```python
from build123d import *

# Parameters (mm, degrees)
BOSS_EXTRU_1_OUTLINE_R = 5
BOSS_EXTRU_1_DEPTH     = 5
CONG_2_R               = 10
CONG_3_R               = 5


# Read off the part's stored shape, not the designer's step: Boss.-Extru.1
with BuildPart() as part:
    # Boss.-Extru.1 outline → Boss.-Extru.1 (new body)
    with BuildSketch(Plane.XY):
        with BuildLine():
            Line((111.825417275, 56.670302216), (105.808192277, 57.923261539))
            ThreePointArc((105.808192277, 57.923261539), (103.288971945, 61.767546768), (107.133257174, 64.2867671))
            Line((107.133257174, 64.2867671), (113.037155155, 63.057405721))
            Line((113.037155155, 63.057405721), (115.346853986, 64.014114302))
            Line((115.346853986, 64.014114302), (111.520019662, 73.252909628))
            Line((111.520019662, 73.252909628), (91.607534943, 56.252195883))
            Line((91.607534943, 56.252195883), (84.536467131, 63.323263695))
            Line((84.536467131, 63.323263695), (82.768700178, 61.555496742))
            Line((82.768700178, 61.555496742), (81.64515805, 55.630550004))
            ThreePointArc((81.64515805, 55.630550004), (77.846557681, 53.042957448), (75.258965125, 56.841557817))
            Line((75.258965125, 56.841557817), (76.404073966, 62.880235609))
            Line((76.404073966, 62.880235609), (59.03555307, 80.248756505))
            Line((59.03555307, 80.248756505), (63.323263695, 84.536467131))
            Line((63.323263695, 84.536467131), (56.252195883, 91.607534943))
            ThreePointArc((56.252195883, 91.607534943), (41.138468979, 99.317049745), (25, 104.552618332))
            Line((25, 104.552618332), (15, 104.552618332))
            Line((15, 104.552618332), (15, 102.052618332))
            Line((15, 102.052618332), (18.395105759, 97.068584057))
            ThreePointArc((18.395105759, 97.068584057), (17.538793922, 92.552863734), (13.023073599, 93.40917557))
            Line((13.023073599, 93.40917557), (9.56279781, 98.488879813))
            Line((9.56279781, 98.488879813), (-15, 98.488879813))
            Line((-15, 98.488879813), (-15, 104.552618332))
            Line((-15, 104.552618332), (-25, 104.552618332))
            ThreePointArc((-25, 104.552618332), (-41.138468979, 99.317049745), (-56.252195883, 91.607534943))
            Line((-56.252195883, 91.607534943), (-63.323263695, 84.536467131))
            Line((-63.323263695, 84.536467131), (-61.555496742, 82.768700178))
            Line((-61.555496742, 82.768700178), (-55.630550004, 81.64515805))
            ThreePointArc((-55.630550004, 81.64515805), (-53.042957448, 77.846557681), (-56.841557817, 75.258965125))
            Line((-56.841557817, 75.258965125), (-62.880235609, 76.404073966))
            Line((-62.880235609, 76.404073966), (-80.248756505, 59.03555307))
            Line((-80.248756505, 59.03555307), (-84.536467131, 63.323263695))
            Line((-84.536467131, 63.323263695), (-91.607534943, 56.252195883))
            ThreePointArc((-91.607534943, 56.252195883), (-99.317049745, 41.138468979), (-104.552618332, 25))
            Line((-104.552618332, 25), (-104.552618332, 15))
            Line((-104.552618332, 15), (-102.052618332, 15))
            Line((-102.052618332, 15), (-97.068584057, 18.395105759))
            ThreePointArc((-97.068584057, 18.395105759), (-92.552863734, 17.538793922), (-93.40917557, 13.023073599))
            Line((-93.40917557, 13.023073599), (-98.488879813, 9.56279781))
            Line((-98.488879813, 9.56279781), (-98.488879813, -15))
            Line((-98.488879813, -15), (-104.552618332, -15))
            Line((-104.552618332, -15), (-104.552618332, -25))
            Line((-104.552618332, -25), (-130.65419128, -27.058933002))
            Line((-130.65419128, -27.058933002), (-126.827356957, -36.297728327))
            Line((-126.827356957, -36.297728327), (-124.517658126, -35.341019746))
            Line((-124.517658126, -35.341019746), (-121.212261595, -30.297043681))
            ThreePointArc((-121.212261595, -30.297043681), (-116.712583661, -29.360081308), (-115.775621287, -33.859759242))
            Line((-115.775621287, -33.859759242), (-119.144465853, -39.000555875))
            Line((-119.144465853, -39.000555875), (-109.744690078, -61.693622033))
            Line((-109.744690078, -61.693622033), (-115.346853986, -64.014114302))
            Line((-115.346853986, -64.014114302), (-111.520019662, -73.252909628))
            Line((-111.520019662, -73.252909628), (-91.607534943, -56.252195883))
            Line((-91.607534943, -56.252195883), (-84.536467131, -63.323263695))
            Line((-84.536467131, -63.323263695), (-82.768700178, -61.555496742))
            Line((-82.768700178, -61.555496742), (-81.64515805, -55.630550004))
            ThreePointArc((-81.64515805, -55.630550004), (-77.846557681, -53.042957448), (-75.258965125, -56.841557817))
            Line((-75.258965125, -56.841557817), (-76.404073966, -62.880235609))
            Line((-76.404073966, -62.880235609), (-59.03555307, -80.248756505))
            Line((-59.03555307, -80.248756505), (-63.323263695, -84.536467131))
            Line((-63.323263695, -84.536467131), (-56.252195883, -91.607534943))
            ThreePointArc((-56.252195883, -91.607534943), (-41.138468979, -99.317049745), (-25, -104.552618332))
            Line((-25, -104.552618332), (-15, -104.552618332))
            Line((-15, -104.552618332), (-15, -102.052618332))
            Line((-15, -102.052618332), (-18.395105759, -97.068584057))
            ThreePointArc((-18.395105759, -97.068584057), (-17.538793922, -92.552863734), (-13.023073599, -93.40917557))
            Line((-13.023073599, -93.40917557), (-9.56279781, -98.488879813))
            Line((-9.56279781, -98.488879813), (15, -98.488879813))
            Line((15, -98.488879813), (15, -104.552618332))
            Line((15, -104.552618332), (25, -104.552618332))
            ThreePointArc((25, -104.552618332), (41.138468979, -99.317049745), (56.252195883, -91.607534943))
            Line((56.252195883, -91.607534943), (63.323263695, -84.536467131))
            Line((63.323263695, -84.536467131), (61.555496742, -82.768700178))
            Line((61.555496742, -82.768700178), (55.630550004, -81.64515805))
            ThreePointArc((55.630550004, -81.64515805), (53.042957448, -77.846557681), (56.841557817, -75.258965125))
            Line((56.841557817, -75.258965125), (62.880235609, -76.404073966))
            Line((62.880235609, -76.404073966), (80.248756505, -59.03555307))
            Line((80.248756505, -59.03555307), (84.536467131, -63.323263695))
            Line((84.536467131, -63.323263695), (91.607534943, -56.252195883))
            ThreePointArc((91.607534943, -56.252195883), (99.317049745, -41.138468979), (104.552618332, -25))
            Line((104.552618332, -25), (104.552618332, -15))
            Line((104.552618332, -15), (102.052618332, -15))
            Line((102.052618332, -15), (97.068584057, -18.395105759))
            ThreePointArc((97.068584057, -18.395105759), (92.552863734, -17.538793922), (93.40917557, -13.023073599))
            Line((93.40917557, -13.023073599), (98.488879813, -9.56279781))
            Line((98.488879813, -9.56279781), (98.488879813, 15))
            Line((98.488879813, 15), (104.552618332, 15))
            Line((104.552618332, 15), (104.552618332, 25))
            Line((104.552618332, 25), (130.65419128, 27.058933002))
            Line((130.65419128, 27.058933002), (126.827356957, 36.297728327))
            Line((126.827356957, 36.297728327), (121.225193049, 33.977236058))
            Line((121.225193049, 33.977236058), (111.825417275, 56.670302216))
        make_face()
        with Locations((-92.387953251, -38.268343237)):
            Circle(BOSS_EXTRU_1_OUTLINE_R, mode=Mode.SUBTRACT)
        with BuildLine():
            ThreePointArc((-2.061552813, -83.5), (-3.811893422, -85.108458961), (-4.498511999, -87.384285714))
            ThreePointArc((-4.498511999, -87.384285714), (-61.871843354, -61.871843354), (-87.384285714, -4.498511999))
            ThreePointArc((-87.384285714, -4.498511999), (-85.108458961, -3.811893422), (-83.5, -2.061552813))
            Line((-83.5, -2.061552813), (-83.5, 2.061552813))
            ThreePointArc((-83.5, 2.061552813), (-85.108458961, 3.811893422), (-87.384285714, 4.498511999))
            ThreePointArc((-87.384285714, 4.498511999), (-61.871843354, 61.871843354), (-4.498511999, 87.384285714))
            ThreePointArc((-4.498511999, 87.384285714), (-3.811893422, 85.108458961), (-2.061552813, 83.5))
            Line((-2.061552813, 83.5), (2.061552813, 83.5))
            ThreePointArc((2.061552813, 83.5), (3.811893422, 85.108458961), (4.498511999, 87.384285714))
            ThreePointArc((4.498511999, 87.384285714), (61.871843354, 61.871843354), (87.384285714, 4.498511999))
            ThreePointArc((87.384285714, 4.498511999), (85.108458961, 3.811893422), (83.5, 2.061552813))
            Line((83.5, 2.061552813), (83.5, -2.061552813))
            ThreePointArc((83.5, -2.061552813), (85.108458961, -3.811893422), (87.384285714, -4.498511999))
            ThreePointArc((87.384285714, -4.498511999), (61.871843354, -61.871843354), (4.498511999, -87.384285714))
            ThreePointArc((4.498511999, -87.384285714), (3.811893422, -85.108458961), (2.061552813, -83.5))
            Line((2.061552813, -83.5), (-2.061552813, -83.5))
        make_face(mode=Mode.SUBTRACT)
        with Locations((92.387953251, 38.268343237)):
            Circle(BOSS_EXTRU_1_OUTLINE_R, mode=Mode.SUBTRACT)
    extrude(amount=BOSS_EXTRU_1_DEPTH)

    # Congé2
    cong_2_edges = [part.edges().sort_by_distance(p)[0] for p in [
        (104.552618332, 25, 2.5),
        (-91.607534943, -56.252195883, 2.5),
        (-104.552618332, -25, 2.5),
        (91.607534943, 56.252195883, 2.5),
    ]]
    fillet(cong_2_edges, radius=CONG_2_R)

    # Congé3
    cong_3_edges = [part.edges().sort_by_distance(p)[0] for p in [
        (130.65419128, 27.058933002, 2.5),
        (-111.520019662, -73.252909628, 2.5),
        (-130.65419128, -27.058933002, 2.5),
        (111.520019662, 73.252909628, 2.5),
    ]]
    fillet(cong_3_edges, radius=CONG_3_R)


solid = part.part
```
Geometry: final body of the model. Coordinates: model frame, mm. A direction names the side the tool comes from. Round coordinates to 2 decimals unless told otherwise and drop trailing zeros. Order: outer loops, then holes, each group sorted by start corner. A loop starts at its lowest first (then second) coordinate and runs counter-clockwise, first axis right, second up. Notation, with made-up numbers: (57, 76.25) - (61, 76.25) arc R11 ccw to (61, 89.25) - close; hole circle Ø7 at (17.5, 39). An arc over 180 degrees is marked (long way). Use CSV: the item, a comma, the result in double quotes. Start each with the question number.
Q1. Section query A-A (x = -40). Return loops of the section in (y, z).
Q2. Access query for faces 4 (the face through (67.841, 71.443, 2.465)), 5 (the face through (110.765, 69.829, 2.535)), 6 (the face through (58.634, -82.215, 2.465)), 7 (the face through (-11.32, -95.91, 2.46)), 8 (the face through (99.226, -41.358, 2.465)). Directions: +Z, -Z, +X, -X, +Y, -Y. A direction counts if a zero-diameter tool reaches every point of the face in a straight line with its end or side. Return the directions, or none.
Q3. Material intervals for line 1 along X through (y, z) = (-18.5, 2.45); line 2 along X through (y, z) = (36.5, 2.8); line 3 along X through (y, z) = (-36, 2.55), sorted ascending. Write a range as from..to.
Q4. Mould query, pull axis Y, two halves, no side actions, for faces 1 (the face through (11.32, 95.91, 2.46)), 2 (the face through (-122.888, -32.854, 2.465)), 3 (the face through (-77.92, -53.03, 2.46)). Classes: +Y half, -Y half, draft (parallel to the pull), parting line (faces both ways), or undercut.
Q5. Section query B-B (x = 66.5). Return loops of the section in (y, z), and give its area (3 significant figures).
Q6. First-contact query: pin 1 (6 mm diameter, centred on x = -92.39, y = -38.27, fed in from -Z); pin 2 (1.5 mm diameter, centred on y = 19, z = 2, fed in from +X); pin 3 (2 mm diameter, centred on x = 0, z = 1.5, fed in from +Y); pin 4 (2 mm diameter, centred on x = -103.5, z = 2.5, fed in from -Y). Flat tips, straight axial feed; report the tip coordinate or a pass-through.
Q7. Section query C-C (z = 1.05). State how many separate pieces and enclosed holes the cut face has, and give its area (3 significant figures).
Result set:
1,outline,"(-99.78, 0) - (-77.82, 0) - (-77.82, 5) - (-99.78, 5) - close; (77.82, 0) - (99.78, 0) - (99.78, 5) - (77.82, 5) - close"
2,face 4,"+Z, -Z"
2,face 5,"+Z, -Z, +Y"
2,face 6,"+Z, -Z, +X"
2,face 7,"+Z, -Z, -Y"
2,face 8,"+Z, -Z, +X, -Y"
3,line 1,"x = -104.94..-85.52, 85.52..93.57, 96.9..104.55"
3,line 2,"x = -101.11..-79.52, 79.52..87.71, 97.06..120.18"
3,line 3,"x = -126.95..-126.11, -117.18..-96.84, -87.93..-79.75, 79.75..101.29"
4,face 1,"+Y half"
4,face 2,"-Y half"
4,face 3,"undercut"
5,outline,"(-72.78, 0) - (-56.87, 0) - (-56.87, 5) - (-72.78, 5) - close; (56.87, 0) - (72.78, 0) - (72.78, 5) - (56.87, 5) - close"
5,area,"159 mm2"
6,pin 1,"passes through"
6,pin 2,"stops at x = 105.38"
6,pin 3,"stops at y = 98.49"
6,pin 4,"stops at y = -67.26"
7,separate pieces,"1"
7,enclosed holes,"3"
7,area,"11,200 mm2"
